from build123d import *

# Parameters (mm, degrees)
SKETCH_1_W      = 12
SKETCH_1_H      = 10
SKETCH_1_R      = 1.35
SKETCH_1_R_2    = 0.7
EXTRUDE_1_DEPTH = 1


with BuildPart() as part:
    # 草图1 → 凸台-拉伸1 (new body)
    with BuildSketch(Plane(origin=(0, 0, 0), x_dir=(1, 0, 0), z_dir=(0, 1, 0))):
        Rectangle(SKETCH_1_W, SKETCH_1_H)
        with Locations(Location((0, 0, 0), (0, 0, 270))):
            Circle(SKETCH_1_R, mode=Mode.SUBTRACT)
        with Locations(Location((-4.5, 3.5, 0), (0, 0, 270))):
            Circle(SKETCH_1_R_2, mode=Mode.SUBTRACT)
        with Locations(Location((4.5, -3.5, 0), (0, 0, 270))):
            Circle(SKETCH_1_R_2, mode=Mode.SUBTRACT)
        with Locations(Location((4.5, 3.75, 0), (0, 0, 270))):
            Circle(SKETCH_1_R_2, mode=Mode.SUBTRACT)
        with Locations(Location((-4.5, -3.75, 0), (0, 0, 270))):
            Circle(SKETCH_1_R_2, mode=Mode.SUBTRACT)
    extrude(amount=EXTRUDE_1_DEPTH)


solid = part.part
Geometry check sheet. Reference: the model listing, model coordinates, mm. Round coordinates to 2 decimals unless told otherwise and drop trailing zeros. Loops run counter-clockwise (first coordinate to the right, second up) from the corner with the lowest first, then second, coordinate; pieces in that order, holes last. Notation, with made-up numbers: (-31, -34) - (-7, -34) arc R28 ccw to (-7, -16) - close; hole circle Ø3 at (4.25, -11.5). An arc over 180 degrees is marked (long way). Answer as CSV lines item,"result".
(1) Cross-section at A-A, the plane x = 4.5. Enter the section's corners in (y, z), and give its area (3 significant figures).
Output values:
outline,"(0, -5) - (1, -5) - (1, -4.45) - (0, -4.45) - close; (0, -3.05) - (1, -3.05) - (1, 2.8) - (0, 2.8) - close; (0, 4.2) - (1, 4.2) - (1, 5) - (0, 5) - close"
area,"7.20 mm²"
(2) Depth check by flat-ended pin: pin 1 Ø2.5 at (x, z) = (0, 0) entering from -Y. Enter the tip coordinate at first touch or a pass-through.
Output values:
pin 1,"passes through"
(3) Release check for a two-part mould opening along Z. For faces 1 (the face through (-0.1, 0.5, 5)), 2 (the face through (4.5, 0.5, 2.8)), 3 (the face through (-1.4, 0, 1)) record: released by +Z, released by -Z, zero draft, split by the parting line, or undercut.
Output values:
face 1,"released by +Z"
face 2,"undercut"
face 3,"zero draft"
(4) Cross-section at B-B, the plane y = 0.25. Enter the section's corners in (x, z).
Output values:
outline,"(-6, -5) - (6, -5) - (6, 5) - (-6, 5) - close; hole circle Ø1.4 at (-4.5, -3.5); hole circle Ø1.4 at (-4.5, 3.75); hole circle Ø2.7 at (0, 0); hole circle Ø1.4 at (4.5, -3.75); hole circle Ø1.4 at (4.5, 3.5)"
(5) Cross-section at C-C, the plane z = -3.75. Enter the section's corners in (x, y), and give its area (3 significant figures).
Output values:
outline,"(-6, 0) - (-5.15, 0) - (-5.15, 1) - (-6, 1) - close; (-3.85, 0) - (3.8, 0) - (3.8, 1) - (-3.85, 1) - close; (5.2, 0) - (6, 0) - (6, 1) - (5.2, 1) - close"
area,"9.29 mm²"
(6) Cross-section at D-D, the plane x = 0. Enter the section's corners in (y, z).
Output values:
outline,"(0, -5) - (1, -5) - (1, -1.35) - (0, -1.35) - close; (0, 1.35) - (1, 1.35) - (1, 5) - (0, 5) - close"
(7) Material ranges on line 1 along Z through (x, y) = (-4, 0.45); line 2 along Z through (x, y) = (5, 0.35); line 3 along X through (y, z) = (0.7, -4), recorded low to high.
Output values:
line 1,"z = -5 to -3.99, -3.01 to 3.26, 4.24 to 5"
line 2,"z = -5 to -4.24, -3.26 to 3.01, 3.99 to 5"
line 3,"x = -6 to -4.99, -4.01 to 3.85, 5.15 to 6"
